Build history of the part. All positions in model axes, mm. A direction names the side the tool comes from. Round coordinates to 2 decimals unless told otherwise and drop trailing zeros. Write each loop counter-clockwise with the first axis right and the second up, starting at its lowest first coordinate (ties: lowest second). Pieces come first, ordered by that corner, then holes. Notation, with made-up numbers: (-28, -39.75) - (-7, -39.75) arc R29 ccw to (-7, -8.75) - close; hole circle Ø3 at (41, -22.5). An arc over 180 degrees is marked (long way). One line per question, with ' | ' between items.
from build123d import *

# Parameters (mm, degrees)
F0_W     = 25
F0_H     = 18
F1_DEPTH = 1
F0_W_2   = 1
F2_DEPTH = 2.5


with BuildPart() as f1:
    # F0 (on Top) → F1 (new body)
    with BuildSketch(Plane.XY):
        with Locations((-35.655684, 11.245334)):
            Rectangle(F0_W, F0_H)
    extrude(amount=F1_DEPTH)

    # F0 (on Top) → F2 (join)
    with BuildSketch(Plane.XY):
        Polygon((-49.155684, 20.245334), (-48.155684, 20.245334), (-23.155684, 20.245334), (-22.155684, 20.245334), (-22.155684, 21.245334), (-49.155684, 21.245334), align=None)
        Polygon((-23.155684, 2.245334), (-48.155684, 2.245334), (-49.155684, 2.245334), (-49.155684, 1.245334), (-22.155684, 1.245334), (-22.155684, 2.245334), align=None)
        with Locations((-48.655684, 11.245334)):
            Rectangle(F0_W_2, F0_H)
        with Locations((-22.655684, 11.245334)):
            Rectangle(F0_W_2, F0_H)
    extrude(amount=F2_DEPTH)


solid = f1.part
Q1. Saw through at A-A, the plane z = 1.75. List the corners of the cut face in (x, y), then the cut area to 3 significant figures.
Found:
outline: (-49.16, 1.25) - (-22.16, 1.25) - (-22.16, 21.25) - (-49.16, 21.25) - close; hole (-48.16, 2.25) - (-23.16, 2.25) - (-23.16, 20.25) - (-48.16, 20.25) - close | area: 90.0 mm^2
Q2. Drop a flat-ended pin along its axis: pin 1 (6 mm diameter, centred on x = -28.5, y = 14.5, fed in from +Z). Give the stop position or say it passes through.
Found:
pin 1: z = 1
Q3. Pull direction Y, two halves, no side cores. Call faces 3 (the flat face through (-36, 11, 0)), 4 (the flat face through (-48.156, 11, 2)), 5 (the flat face through (-36, 1.245, 1)): +Y half, -Y half, draft (parallel to the pull), parting line (faces both ways), or undercut.
Found:
face 3: draft | face 4: undercut | face 5: -Y half
Q4. Saw through at C-C, the plane x = -25.25. List the corners of the cut face in (y, z).
Found:
outline: (1.25, 0) - (21.25, 0) - (21.25, 2.5) - (20.25, 2.5) - (20.25, 1) - (2.25, 1) - (2.25, 2.5) - (1.25, 2.5) - close
Q5. Drill centre lines: L1, parallel to X at y = 10.25, z = 1.5; L2, parallel to Y at x = -38, z = 1.35; L3, parallel to Z at x = -34.25, y = 18.5. Where is each one in solid material? Low to high. Write a range as from..to.
Found:
L1: -49.16..-48.16, -23.16..-22.16 | L2: 1.25..2.25, 20.25..21.25 | L3: 0..1
Q6. Saw through at B-B, the plane y = 17.75. List the corners of the cut face in (x, z), then the cut area to 3 significant figures.
Found:
outline: (-49.16, 0) - (-22.16, 0) - (-22.16, 2.5) - (-23.16, 2.5) - (-23.16, 1) - (-48.16, 1) - (-48.16, 2.5) - (-49.16, 2.5) - close | area: 30.0 mm^2
Q7. Which spindle directions (+Z, -Z, +X, -X, +Y, -Y) get a long thin tool onto all of the face, cutting with end or side? Do faces 1 (the flat face through (-36, 11, 1)), 2 (the flat face through (-35, 21.245, 1)). Say none if no direction does.
Found:
face 1: +Z | face 2: +Z, -Z, +X, -X, +Y
